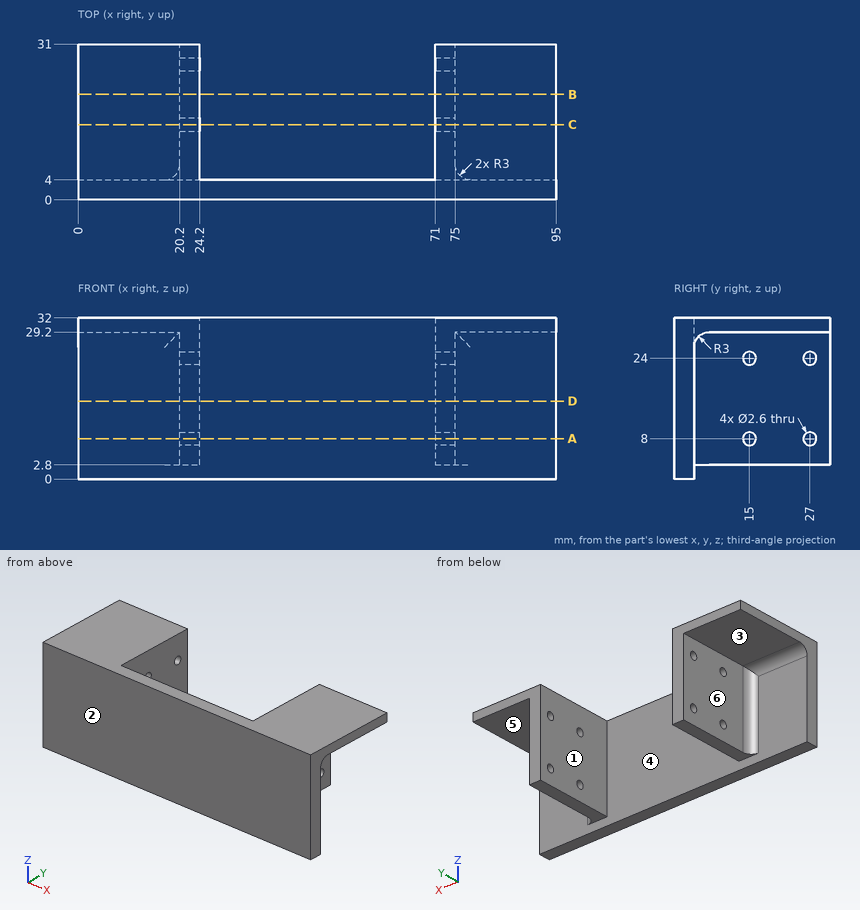
For this review, use the dimensioned drawing (mm, ordinates from the lowest corner) and the shaded views. A direction names the side the tool comes from. Give positions to 0.01 mm unless a question says otherwise; leave off trailing zeros. Write each loop counter-clockwise with the first axis right and the second up, starting at its lowest first coordinate (ties: lowest second). Pieces come first, ordered by that corner, then holes. Notation, with made-up numbers: M 89,-23 L 113,-23 A16 ccw 113,-6 Z; hole C 87,-36 d1. An arc over 180 degrees is marked long. Answer as a JSON object with one key per item and string values. Group by question number.
1) We need section C-C (y = 15). Give the boundary of the cut face in (x, z).
2) Clearance check with flat-ended pins moving along their axes: pin 1 Ø10 at (y, z) = (17, 13.5) entering from -X; pin 2 Ø7.5 at (x, y) = (22, 13) entering from -Z; pin 3 Ø1.5 at (x, z) = (80.5, 9) entering from +Y. State where each tip first meets the part, or that it passes through.
3) Tool access review of the marked faces 1, 2 and 3: name each direction out of +Z, -Z, +X, -X, +Y, -Y from which nothing blocks a thin tool from reaching the whole face with its end or side.
4) We need section B-B (y = 21). Give the boundary of the cut face in (x, z).
5) We need section A-A (z = 8). Count the separate pieces of the cut face and the enclosed holes in it, and give its area (3 significant figures).
6) We need section D-D (z = 15.5). Give the boundary of the cut face in (x, y).
7) Mouldability with a two-part tool opening along X and no side actions: class the marked faces 4, 5 and 6 as released by +X, released by -X, zero draft, split by the parting line, or undercut.
8) For line 1 along Y through (x, z) = (72, 24); line 2 along X through (y, z) = (18, 12); line 3 along Y through (x, z) = (30, 31), list the stretches that pass through material, from the lowest coordinate up.
Answer key:
{
 "1": {"outline": "M 0,29.2 L 20.2,29.2 L 20.2,25.3 L 24.2,25.3 L 24.2,32 L 0,32 Z; M 20.2,2.8 L 24.2,2.8 L 24.2,6.7 L 20.2,6.7 Z; M 20.2,9.3 L 24.2,9.3 L 24.2,22.7 L 20.2,22.7 Z; M 71,2.8 L 75,2.8 L 75,6.7 L 71,6.7 Z; M 71,9.3 L 75,9.3 L 75,22.7 L 71,22.7 Z; M 71,25.3 L 75,25.3 L 75,29.2 L 95,29.2 L 95,32 L 71,32 Z"},
 "2": {"pin 1": "stops at x = 20.2", "pin 2": "stops at z = 2.8", "pin 3": "stops at y = 4"},
 "3": {"face 1": "+Z, -Z, +Y", "face 2": "+Z, -Z, +X, -X, -Y", "face 3": "-Z, -X, +Y"},
 "4": {"outline": "M 0,29.2 L 20.2,29.2 L 20.2,2.8 L 24.2,2.8 L 24.2,32 L 0,32 Z; M 71,2.8 L 75,2.8 L 75,29.2 L 95,29.2 L 95,32 L 71,32 Z"},
 "5": {"separate pieces": "5", "enclosed holes": "0", "area": "558 mm²"},
 "6": {"outline": "M 0,0 L 95,0 L 95,4 L 78,4 A3 cw 75,7 L 75,31 L 71,31 L 71,4 L 24.2,4 L 24.2,31 L 20.2,31 L 20.2,7 A3 cw 17.2,4 L 0,4 Z"},
 "7": {"face 4": "undercut", "face 5": "zero draft", "face 6": "released by -X"},
 "8": {"line 1": "y = 0 to 13.7, 16.3 to 25.7, 28.3 to 31", "line 2": "x = 20.2 to 24.2, 71 to 75", "line 3": "y = 0 to 4"}
}
